Read the model definition and answer for the solid it produces. Units are mm, in the model's axes. Coordinates: 2 decimals unless noted, no trailing zeros. Loops run counter-clockwise (first coordinate to the right, second up) from the corner with the lowest first, then second, coordinate; pieces in that order, holes last. Notation, with made-up numbers: M -39,87 L -29,87 A10 ccw -29,93 Z; hole C -10.5,-1.75 d2. An arc over 180 degrees is marked long. Use one line per item in the form item = value. Start each with the question number.
1. A flat-ended cylindrical pin translates along its axis: pin 1 (4.5 mm diameter, centred on x = 0, y = 0, fed in from +Z). Find the tip coordinate at first contact, or state that the pin passes through.
2. The part is cut by section D-D (y = -10.5). Give the vertices of the cut face in (x, z), plus the area to 3 significant figures.
3. Find the intervals of material crossed by probe 1 along X at (y, z) = (-15.5, -1.45); probe 2 along Y at (x, z) = (13, -0.55); probe 3 along Y at (x, z) = (-18, -1.8), in increasing order. Write a range as [from, to].
4. The part is cut by section A-A (x = 0). Give the vertices of the cut face in (y, z).
5. The part is cut by section B-B (y = 0). Give the vertices of the cut face in (x, z), plus the area to 3 significant figures.
6. The part is cut by section C-C (z = -0.95). Give the number of separate pieces and of enclosed holes in the cut face, plus the area to 3 significant figures.
7. For a pull along X with two mould halves and no side action, classify faces 1 (the cylindrical face through (1.86, 0.58, -1.36)), 2 (the cylindrical face through (-16.524, -0.064, -1.356)), 3 (the cylindrical face through (16.524, 0.064, -1.356)) as released by +X, released by -X, zero draft, split by the parting line, or undercut.
from build123d import *

# Parameters (mm, degrees)
F0_R            = 19.416407865
F1_DEPTH        = 2.75
F3_DEPTH        = 2.75
F3_COPIES_COUNT = 10
F5_DEPTH        = 25
F5_COPIES_COUNT = 10
F6_R            = 1.9472144129
F7_DEPTH        = 25
F8_R            = 0.5
F9_DEPTH        = 25
F9_COPIES_COUNT = 10


# Not quite as in the source:
# - a pattern or mirror of a feature is missing from the dataset's text; its kind, count and spacing are read off the source's solid


with BuildPart() as f1:
    # F0 (on Top) → F1 (new body)
    with BuildSketch(Plane.XY):
        Circle(F0_R)
    extrude(amount=-F1_DEPTH)

    # F2 (on face) → F3 (join)
    with BuildSketch(Plane.XY):
        with BuildLine():
            ThreePointArc((-2.7430957606, 19.22166278), (0, 19.416407865), (2.7430957606, 19.22166278))
            ThreePointArc((2.7430957606, 19.22166278), (0, 22.166407865), (-2.7430957606, 19.22166278))
        make_face()
    f3 = extrude(amount=-F3_DEPTH)

    # F3_copies: F3 ×10 about axis
    f3_copies_axis = Axis((0, 0, 0), (0, 0, 1))
    for i in range(1, F3_COPIES_COUNT):
        add(f3.rotate(f3_copies_axis, i * 360 / F3_COPIES_COUNT))

    # F4 (on face) → F5 (cut)
    with BuildSketch(Plane.XY):
        with BuildLine():
            Line((-6.2381998898, 19.1992051025), (-9.0789988191, 17.1630030829))
            ThreePointArc((-9.0789988191, 17.1630030829), (-5.1059656467, 15.7145464123), (-2.7430957606, 19.22166278))
            Line((-2.7430957606, 19.22166278), (-6.2381998898, 19.1992051025))
        make_face()
    f5 = extrude(amount=-F5_DEPTH, mode=Mode.SUBTRACT)

    # F5_copies: F5 ×10 about axis
    f5_copies_axis = Axis((0, 0, 0), (0, 0, 1))
    for i in range(1, F5_COPIES_COUNT):
        add(f5.rotate(f5_copies_axis, i * 360 / F5_COPIES_COUNT), mode=Mode.SUBTRACT)

    # F6 (on face) → F7 (cut)
    with BuildSketch(Plane.XY):
        Circle(F6_R)
    extrude(amount=-F7_DEPTH, mode=Mode.SUBTRACT)

    # F8 (on face) → F9 (cut)
    with BuildSketch(Plane.XY):
        with Locations((0, 19.2206762207)):
            Circle(F8_R)
    f9 = extrude(amount=-F9_DEPTH, mode=Mode.SUBTRACT)

    # F9_copies: F9 ×10 about axis
    f9_copies_axis = Axis((0, 0, 0), (0, 0, 1))
    for i in range(1, F9_COPIES_COUNT):
        add(f9.rotate(f9_copies_axis, i * 360 / F9_COPIES_COUNT), mode=Mode.SUBTRACT)


solid = f1.part
Computed values:
q1.pin_1 = 0
q2.outline = M -12.94,-2.75 L 12.94,-2.75 L 12.94,0 L -12.94,0 Z
q2.area = 71.2 mm²
q3.probe_1 = [-14.15, -11.8], [-10.8, 10.8], [11.8, 14.15]
q3.probe_2 = [-17.95, -13.11], [-10.35, 10.35], [13.11, 17.95]
q3.probe_3 = [-8.71, -6.35], [-5.53, -2.82], [2.82, 5.53], [6.35, 8.71]
q4.outline = M -22.17,-2.75 L -19.72,-2.75 L -19.72,0 L -22.17,0 Z; M -18.72,-2.75 L -1.95,-2.75 L -1.95,0 L -18.72,0 Z; M 1.95,-2.75 L 18.72,-2.75 L 18.72,0 L 1.95,0 Z; M 19.72,-2.75 L 22.17,-2.75 L 22.17,0 L 19.72,0 Z
q5.outline = M -16.52,-2.75 L -1.95,-2.75 L -1.95,0 L -16.52,0 Z; M 1.95,-2.75 L 16.52,-2.75 L 16.52,0 L 1.95,0 Z
q5.area = 80.2 mm²
q6.separate_pieces = 1
q6.enclosed_holes = 11
q6.area = 1,150 mm²
q7.face_1 = undercut
q7.face_2 = released by -X
q7.face_3 = released by +X
